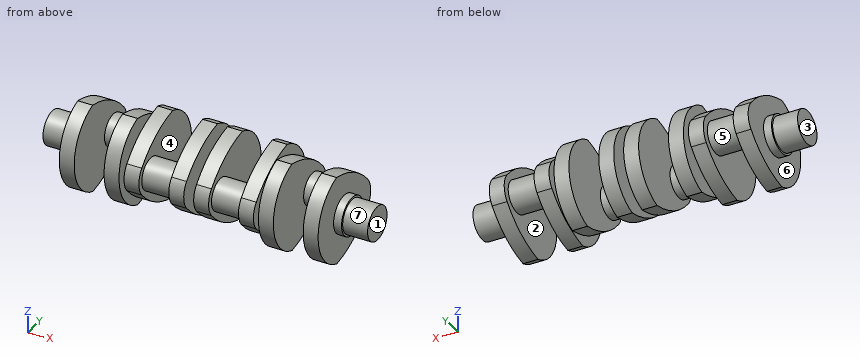
from build123d import *

# Parameters (mm, degrees)
SKETCH1_R            = 17
BOSS_EXTRUDE3_DEPTH  = 25
SKETCH1_5_R          = 19
BOSS_EXTRUDE4_DEPTH  = 8
BOSS_EXTRUDE5_DEPTH  = 15
SKETCH3_R            = 16
BOSS_EXTRUDE6_DEPTH  = 15
MIRROR1_START        = 53
MIRROR1_DEPTH        = 15
MIRROR1_START_2      = 38
MIRROR1_2_OUTLINE_R  = 16
MIRROR1_2_DEPTH      = 15
BOSS_EXTRUDE7_START  = 5
SKETCH4_R            = 17
BOSS_EXTRUDE7_DEPTH  = 5
BOSS_EXTRUDE8_DEPTH  = 15
SKETCH6_R            = 16
BOSS_EXTRUDE9_DEPTH  = 30
BOSS_EXTRUDE10_DEPTH = 15
BOSS_EXTRUDE11_START = 5
SKETCH8_R            = 17
BOSS_EXTRUDE11_DEPTH = 5


# Read off the part's stored shape, not the designer's step: Mirror1
with BuildPart() as part:
    # Sketch1 → Boss-Extrude3 (new body)
    with BuildSketch(Plane(origin=(0, 0, 0), x_dir=(0, 0, -1), z_dir=(1, 0, 0))):
        Circle(SKETCH1_R)
    extrude(amount=-BOSS_EXTRUDE3_DEPTH)

    # Sketch1<5> → Boss-Extrude4 (add)
    with BuildSketch(Plane(origin=(0, 0, 0), x_dir=(0, 0, -1), z_dir=(1, 0, 0))):
        Circle(SKETCH1_5_R)
    extrude(amount=BOSS_EXTRUDE4_DEPTH)

    # Sketch2 → Boss-Extrude5 (add)
    with BuildSketch(Plane(origin=(8, 0, 0), x_dir=(0, 0, -1), z_dir=(1, 0, 0))):
        with BuildLine():
            ThreePointArc((-13.706014257, 40.910536546), (-0.050406066, 45.999939505), (13.629476778, 40.97614981))
            ThreePointArc((13.629476778, 40.97614981), (33.671459186, 16.608703248), (44.071795254, -13.178651794))
            ThreePointArc((44.071795254, -13.178651794), (0.246197834, -45.999341154), (-43.928204746, -13.649645701))
            ThreePointArc((-43.928204746, -13.649645701), (-33.694579877, 16.332192974), (-13.706014257, 40.910536546))
        make_face()
    extrude(amount=BOSS_EXTRUDE5_DEPTH)

    # Sketch3 → Boss-Extrude6 (add)
    with BuildSketch(Plane(origin=(23, 0, 0), x_dir=(0, 0, -1), z_dir=(1, 0, 0))):
        with Locations((-0.025203033, 22.999969753)):
            Circle(SKETCH3_R)
    extrude(amount=BOSS_EXTRUDE6_DEPTH)



with BuildPart() as body_2:
    # Mirror1 outline → Mirror1 (new body)
    with BuildSketch(Plane.YZ.offset(MIRROR1_START)):
        with BuildLine():
            ThreePointArc((40.97614981, -13.629476778), (45.999939505, 0.050406066), (40.910536546, 13.706014257))
            ThreePointArc((40.910536546, 13.706014257), (16.332192974, 33.694579877), (-13.649645701, 43.928204746))
            ThreePointArc((-13.649645701, 43.928204746), (-45.999341154, -0.246197834), (-13.178651794, -44.071795254))
            ThreePointArc((-13.178651794, -44.071795254), (16.608703248, -33.671459186), (40.97614981, -13.629476778))
        make_face()
    extrude(amount=MIRROR1_DEPTH)


with BuildPart() as part_1:
    add(part.part)

    add(body_2.part)  # Mirror1 2 merges body 2
    # Mirror1 2 outline → Mirror1 2 (add)
    with BuildSketch(Plane.YZ.offset(MIRROR1_START_2)):
        with Locations((22.999969753, 0.025203033)):
            Circle(MIRROR1_2_OUTLINE_R)
    extrude(amount=MIRROR1_2_DEPTH)

    # Sketch4 → Boss-Extrude7 (add)
    with BuildSketch(Plane(origin=(68, 0, 0), x_dir=(0, 0, -1), z_dir=(1, 0, 0)).offset(BOSS_EXTRUDE7_START)):
        Circle(SKETCH4_R)
    extrude(amount=-BOSS_EXTRUDE7_DEPTH)

    # Sketch5 → Boss-Extrude8 (add)
    with BuildSketch(Plane(origin=(73, 0, 0), x_dir=(0, 0, -1), z_dir=(1, 0, 0))):
        with BuildLine():
            ThreePointArc((-13.629476778, -40.97614981), (0.050406066, -45.999939505), (13.706014257, -40.910536546))
            ThreePointArc((13.706014257, -40.910536546), (33.694579877, -16.332192974), (43.928204746, 13.649645701))
            ThreePointArc((43.928204746, 13.649645701), (-0.246197834, 45.999341154), (-44.071795254, 13.178651794))
            ThreePointArc((-44.071795254, 13.178651794), (-33.671459186, -16.608703248), (-13.629476778, -40.97614981))
        make_face()
    extrude(amount=BOSS_EXTRUDE8_DEPTH)

    # Sketch6 → Boss-Extrude9 (add)
    with BuildSketch(Plane(origin=(88, 0, 0), x_dir=(0, 0, -1), z_dir=(1, 0, 0))):
        with Locations((0, -25)):
            Circle(SKETCH6_R)
    extrude(amount=BOSS_EXTRUDE9_DEPTH)

    # Sketch7 → Boss-Extrude10 (add)
    with BuildSketch(Plane(origin=(118, 0, 0), x_dir=(0, 0, -1), z_dir=(1, 0, 0))):
        with BuildLine():
            ThreePointArc((-13.629476778, -40.97614981), (0.050406066, -45.999939505), (13.706014257, -40.910536546))
            ThreePointArc((13.706014257, -40.910536546), (33.694579877, -16.332192974), (43.928204746, 13.649645701))
            ThreePointArc((43.928204746, 13.649645701), (-0.246197834, 45.999341154), (-44.071795254, 13.178651794))
            ThreePointArc((-44.071795254, 13.178651794), (-33.671459186, -16.608703248), (-13.629476778, -40.97614981))
        make_face()
    extrude(amount=BOSS_EXTRUDE10_DEPTH)

    # Sketch8 → Boss-Extrude11 (add)
    with BuildSketch(Plane(origin=(133, 0, 0), x_dir=(0, 0, -1), z_dir=(1, 0, 0)).offset(BOSS_EXTRUDE11_START)):
        Circle(SKETCH8_R)
    extrude(amount=-BOSS_EXTRUDE11_DEPTH)

    # Mirror2: part across plane


with BuildPart() as part_2:
    add(part_1.part)
    add(part_1.part.mirror(Plane(origin=(138, 0, 0), x_dir=(0, 0, 1), z_dir=(1, 0, 0))))


solid = part_2.part
Work out the finished part from the listing and answer in its coordinate system (mm). Face numbers are marked on the shaded views. A direction names the side the tool comes from. Coordinates: 2 decimals unless noted, no trailing zeros. Write each loop counter-clockwise with the first axis right and the second up, starting at its lowest first coordinate (ties: lowest second). Pieces come first, ordered by that corner, then holes. Notation, with made-up numbers: M -19.75,88 L 39.25,88 A31 cw 39.25,117 Z; hole C 38,19 d11. An arc over 180 degrees is marked long. Use one line per item in the form item = value. Start each with the question number.
1. Straight lines are drawn through the part: probe 1 along X at (y, z) = (-22, 10); probe 2 along X at (y, z) = (34.5, -8); probe 3 along X at (y, z) = (28.5, 27.5). For each, find the intervals that lie inside material, in ascending order. Write a range as from..to.
2. The part is cut by section B-B (x = 121). Give the vertices of the cut face in (y, z), plus the area to 3 significant figures.
3. A tool of negligible diameter and unlimited length cuts with its end or side. For the marked faces 5, 6 and 7, from which of +Z, -Z, +X, -X, +Y, -Y can it reach the whole face along a straight path? Write none if from no direction.
4. The part is cut by section C-C (y = 0). Give the number of separate pieces and of enclosed holes in the cut face, plus the area to 3 significant figures.
5. Each of these flat-tipped pins is pushed along its axis until it touches: P1, Ø10, axis at y = 36.5, z = -27.5, coming from the +X side; P2, Ø6, axis at x = 127, z = 16.5, coming from the +Y side; P3, Ø6, axis at x = 268.5, y = 22, coming from the +Z side. Where does it stop, or does it pass through?
6. The mould has two halves that part along X. Classify the marked faces 1, 2, 3 and 4: released by +X, released by -X, zero draft, split by the parting line, or undercut.
Evaluation:
q1.probe_1 = 8..23, 53..68, 73..133, 143..203, 208..223, 253..268
q1.probe_2 = 8..68, 73..88, 118..133, 143..158, 188..203, 208..268
q1.probe_3 = 73..88, 118..133, 143..158, 188..203
q2.outline = M -40.98,13.63 A21 ccw -40.91,-13.71 A90 ccw 13.65,-43.93 A46 ccw 13.18,44.07 A90 ccw Z
q2.area = 5,800 mm^2
q3.face_5 = none
q3.face_6 = -X
q3.face_7 = +X
q4.separate_pieces = 5
q4.enclosed_holes = 0
q4.area = 12,800 mm^2
q5.P1 = 203
q5.P2 = 43.97
q5.P3 = 32.13
q6.face_1 = released by +X
q6.face_2 = undercut
q6.face_3 = released by -X
q6.face_4 = undercut
